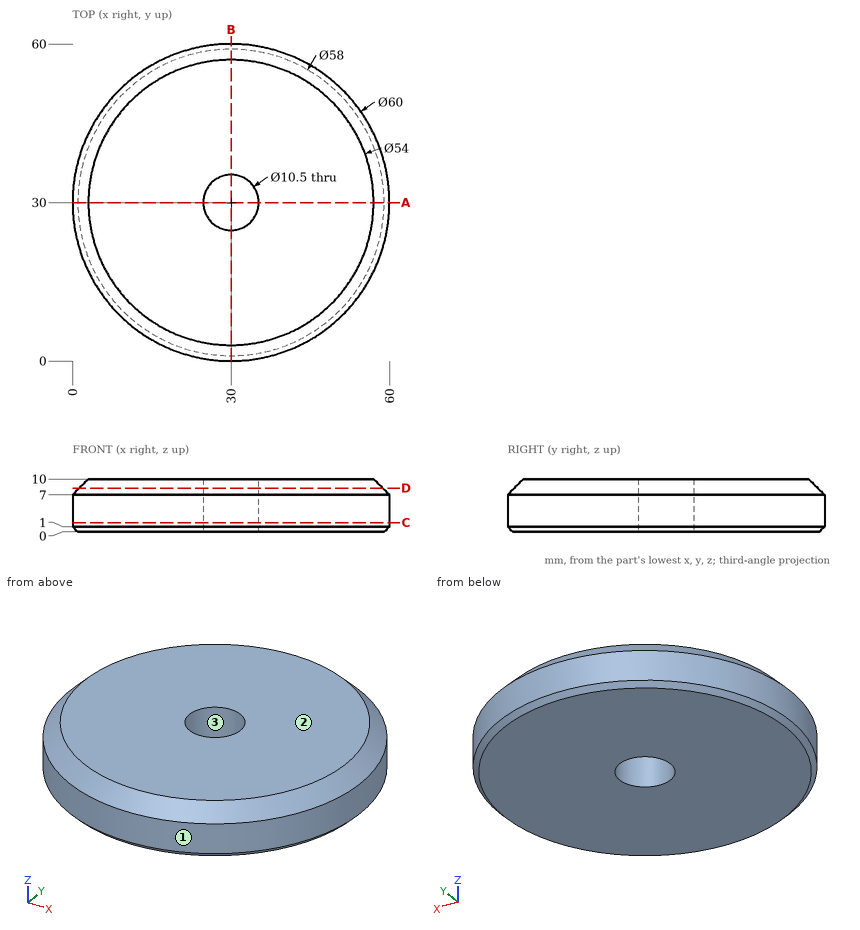
For this review, use the dimensioned drawing (mm, ordinates from the lowest corner) and the shaded views. Coordinates: 2 decimals unless noted, no trailing zeros. Loops run counter-clockwise (first coordinate to the right, second up) from the corner with the lowest first, then second, coordinate; pieces in that order, holes last. Notation, with made-up numbers: (55.5, 15.25) - (72.5, 15.25) arc R21 ccw to (72.5, 29.25) - close; hole circle Ø11 at (68.5, 78.25). An arc over 180 degrees is marked (long way). Use one line per item in the form item = value. Start each with the question number.
1) To check wall thickness, follow probe 1 along Y at (x, z) = (30, 4.75); probe 2 along Y at (x, z) = (31.5, 8.5); probe 3 along X at (y, z) = (30.5, 1.25). State the ranges of each line that lie inside material, in increasing order. Write a range as from..to.
2) Take a section at C-C (z = 1.75). State the section outline as (x, y) points.
3) Draft analysis for pull direction Y (two halves, no side actions). For the marked faces 1, 2 and 3, state which applies: released by +Y, released by -Y, zero draft, split by the parting line, or undercut.
4) Take a section at D-D (z = 8.25). State the section outline as (x, y) points, plus the area to 3 significant figures.
5) Take a section at A-A (y = 30). State the section outline as (x, z) points.
6) For pin 1 (3 mm diameter, centred on x = 20.5, z = 7, fed in from -Y); pin 2 (1.5 mm diameter, centred on y = 11.5, z = 6, fed in from +X); pin 3 (4 mm diameter, centred on x = 20.5, z = 1, fed in from -Y); pin 4 (5 mm diameter, centred on x = 53.5, y = 47, fed in from +Z), all flat-tipped, find the tip position at first contact; note any pin that passes through.
From the geometry:
q1.probe_1 = 0..24.75, 35.25..60
q1.probe_2 = 1.54..24.97, 35.03..58.46
q1.probe_3 = 0..24.77, 35.23..60
q2.outline = circle Ø60 at (30, 30); hole circle Ø10.5 at (30, 30)
q3.face_1 = split by the parting line
q3.face_2 = zero draft
q3.face_3 = undercut
q4.outline = circle Ø57.5 at (30, 30); hole circle Ø10.5 at (30, 30)
q4.area = 2,510 mm2
q5.outline = (0, 1) - (1, 0) - (24.75, 0) - (24.75, 10) - (3, 10) - (0, 7) - close; (35.25, 0) - (59, 0) - (60, 1) - (60, 7) - (57, 10) - (35.25, 10) - close
q6.pin_1 = 1.09
q6.pin_2 = 54.19
q6.pin_3 = 0.95
q6.pin_4 = 10
